The listing builds one solid part. Answer for the finished solid, in the listing's coordinates (mm). Coordinates: 2 decimals unless noted, no trailing zeros. Order: outer loops, then holes, each group sorted by start corner. A loop starts at its lowest first (then second) coordinate and runs counter-clockwise, first axis right, second up. Notation, with made-up numbers: (81, 86.25) - (134, 86.25) arc R27 cw to (134, 104.25) - close; hole circle Ø4 at (52, -3). An arc over 180 degrees is marked (long way). Use a Markdown table: item, result. Add a question column.
Item 1: The part is cut by section B-B, the plane y = -38.5. Give the vertices of the cut face in (x, z).
Item 2: A flat-ended cylindrical pin translates along its axis: P1, Ø3.5, axis at x = 17.5, y = -38.5, coming from the +Z side. Find the tip coordinate at first contact, or state that the pin passes through.
Item 3: The part is cut by section C-C, the plane x = -17.5. Give the vertices of the cut face in (y, z).
Item 4: The part is cut by section A-A, the plane z = 3.2. State how many separate pieces and enclosed holes the cut face has, then the cut area to 3 significant figures.
Item 5: Find the intervals of material crossed by line 1 along Y through (x, z) = (-17.5, 2.5); line 2 along Y through (x, z) = (0, 2.9); line 3 along X through (y, z) = (39.5, 0.65), in increasing order.
from build123d import *

# Parameters (mm, degrees)
ESQUISSE1_W        = 55
ESQUISSE1_H        = 85
BOSS_EXTRU_1_DEPTH = 5
SKETCH1_R          = 2
CUT_EXTRUDE1_DEPTH = 10
CUT_EXTRUDE2_START = -10
CUT_EXTRUDE2_DEPTH = 10
SKETCH3_R          = 2.5
CUT_EXTRUDE3_DEPTH = 10


with BuildPart() as part:
    # Esquisse1 → Boss.-Extru.1 (new body)
    with BuildSketch(Plane.XY):
        Rectangle(ESQUISSE1_W, ESQUISSE1_H)
    extrude(amount=BOSS_EXTRU_1_DEPTH)

    # Sketch1 → Cut-Extrude1 (cut)
    with BuildSketch(Plane.XY.offset(5)):
        with Locations((-17.5, 38.5)):
            Circle(SKETCH1_R)
        with Locations((-17.5, 7.5)):
            Circle(SKETCH1_R)
        with Locations(Location((17.5, 7.5, 0), (0, 0, 180))):
            Circle(SKETCH1_R)
        with Locations(Location((17.5, 38.5, 0), (0, 0, 180))):
            Circle(SKETCH1_R)
        with Locations((17.5, -38.5)):
            Circle(SKETCH1_R)
        with Locations((17.5, -7.5)):
            Circle(SKETCH1_R)
        with Locations(Location((-17.5, -7.5, 0), (0, 0, 180))):
            Circle(SKETCH1_R)
        with Locations(Location((-17.5, -38.5, 0), (0, 0, 180))):
            Circle(SKETCH1_R)
    extrude(amount=-CUT_EXTRUDE1_DEPTH, mode=Mode.SUBTRACT)

    # Sketch2 → Cut-Extrude2 (cut)
    with BuildSketch(Plane(origin=(0, 0, 0), x_dir=(-1, 0, 0), z_dir=(0, 0, -1)).offset(CUT_EXTRUDE2_START)):
        with BuildLine():
            Line((-19.5, 7.5), (-19.5, 5.5))
            ThreePointArc((-19.5, 5.5), (-17.5, 3.5), (-15.5, 5.5))
            Line((-15.5, 5.5), (-15.5, 7.5))
            ThreePointArc((-15.5, 7.5), (-17.5, 9.5), (-19.5, 7.5))
        make_face()
        with BuildLine():
            Line((15.5, 7.5), (15.5, 5.5))
            ThreePointArc((15.5, 5.5), (17.5, 3.5), (19.5, 5.5))
            Line((19.5, 5.5), (19.5, 7.5))
            ThreePointArc((19.5, 7.5), (17.5, 9.5), (15.5, 7.5))
        make_face()
        with BuildLine():
            Line((19.5, -7.5), (19.5, -5.5))
            ThreePointArc((19.5, -5.5), (17.5, -3.5), (15.5, -5.5))
            Line((15.5, -5.5), (15.5, -7.5))
            ThreePointArc((15.5, -7.5), (17.5, -9.5), (19.5, -7.5))
        make_face()
        with BuildLine():
            Line((-15.5, -7.5), (-15.5, -5.5))
            ThreePointArc((-15.5, -5.5), (-17.5, -3.5), (-19.5, -5.5))
            Line((-19.5, -5.5), (-19.5, -7.5))
            ThreePointArc((-19.5, -7.5), (-17.5, -9.5), (-15.5, -7.5))
        make_face()
    extrude(amount=CUT_EXTRUDE2_DEPTH, mode=Mode.SUBTRACT)

    # Sketch3 → Cut-Extrude3 (cut)
    with BuildSketch(Plane.XY.offset(5)):
        Circle(SKETCH3_R)
    extrude(amount=-CUT_EXTRUDE3_DEPTH, mode=Mode.SUBTRACT)


solid = part.part
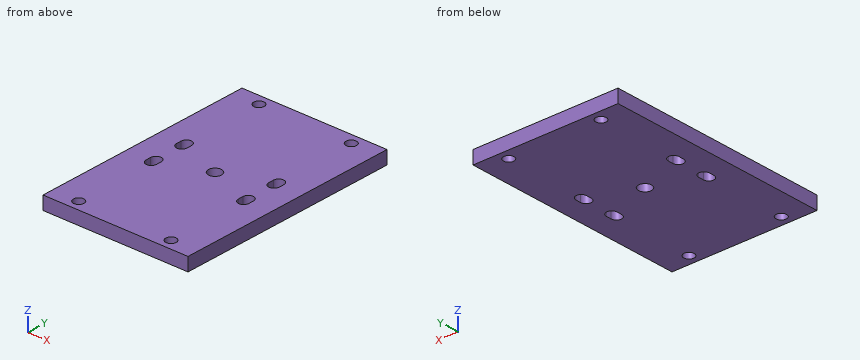
Solution:
| question | item | result |
|---|---|---|
| 1 | outline | (-27.5, 0) - (-19.5, 0) - (-19.5, 5) - (-27.5, 5) - close; (-15.5, 0) - (15.5, 0) - (15.5, 5) - (-15.5, 5) - close; (19.5, 0) - (27.5, 0) - (27.5, 5) - (19.5, 5) - close |
| 2 | P1 | passes through |
| 3 | outline | (-42.5, 0) - (-40.5, 0) - (-40.5, 5) - (-42.5, 5) - close; (-36.5, 0) - (-9.5, 0) - (-9.5, 5) - (-36.5, 5) - close; (-3.5, 0) - (3.5, 0) - (3.5, 5) - (-3.5, 5) - close; (9.5, 0) - (36.5, 0) - (36.5, 5) - (9.5, 5) - close; (40.5, 0) - (42.5, 0) - (42.5, 5) - (40.5, 5) - close |
| 4 | separate pieces | 1 |
| 4 | enclosed holes | 9 |
| 4 | area | 4,520 mm2 |
| 5 | line 1 | y = -42.5 to -40.5, -36.5 to -9.5, -3.5 to 3.5, 9.5 to 36.5, 40.5 to 42.5 |
| 5 | line 2 | y = -42.5 to -2.5, 2.5 to 42.5 |
| 5 | line 3 | x = -27.5 to -19.23, -15.77 to 15.77, 19.23 to 27.5 |
